```python
from build123d import *

# Parameters (mm, degrees)
SKETCH1_R           = 65
BOSS_EXTRUDE1_DEPTH = 30
SKETCH2_R           = 50
BOSS_EXTRUDE2_DEPTH = 250
FILLET1_R           = 10
FILLET2_R           = 10
SKETCH3_W           = 60
SKETCH3_H           = 35
BOSS_EXTRUDE3_DEPTH = 65
SKETCH4_R           = 13.35
CUT_EXTRUDE1_DEPTH  = 130
FILLET3_R           = 25


with BuildPart() as part:
    # Sketch1 → Boss-Extrude1 (new body)
    with BuildSketch(Plane(origin=(0, 0, 0), x_dir=(1, 0, 0), z_dir=(0, 1, 0))):
        with Locations(Location((0, 0, 0), (0, 0, 270))):
            Circle(SKETCH1_R)
    extrude(amount=BOSS_EXTRUDE1_DEPTH)

    # Sketch2 → Boss-Extrude2 (add)
    with BuildSketch(Plane.XZ):
        with Locations(Location((0, 0, 0), (0, 0, 90))):
            Circle(SKETCH2_R)
    extrude(amount=BOSS_EXTRUDE2_DEPTH)

    # Fillet1
    fillet1_edges = [part.edges().sort_by_distance(p)[0] for p in [
        (0, 0, -50),
    ]]
    fillet(fillet1_edges, radius=FILLET1_R)

    # Fillet2
    # the kernel refuses this fillet: 10 mm, written as the material it takes off along each edge
    with BuildSketch(Plane(origin=(0, 0, 0), x_dir=(0, 0, 1), z_dir=(-1, 0, 0))) as fillet2_piece_1:
        with BuildLine():
            CenterArc((55, 9.364916731), FILLET2_R, 284.477512186, 75.522487814)
            Line((65, 9.364916731), (66, 9.364916731))
            Line((66, 9.364916731), (66, 0))
            Line((66, 0), (65, -1))
            ThreePointArc((65, -1), (60, -1), (57.75, -1.285787471))
            Line((57.75, -1.285787471), (57.5, -0.317541634))
        make_face()
    revolve(axis=Axis((0, 0, 0), (0, 1, 0)), mode=Mode.SUBTRACT)

    # Sketch3 → Boss-Extrude3 (add, symmetric)
    with BuildSketch(Plane(origin=(0, 0, 0), x_dir=(0, 0, -1), z_dir=(1, 0, 0))):
        with Locations((0, 47.5)):
            Rectangle(SKETCH3_W, SKETCH3_H)
    extrude(amount=BOSS_EXTRUDE3_DEPTH, both=True)

    # Sketch4 → Cut-Extrude1 (cut)
    with BuildSketch(Plane(origin=(65, 0, 0), x_dir=(0, 0, -1), z_dir=(1, 0, 0))):
        with Locations((0, 47.897467929)):
            Circle(SKETCH4_R)
    extrude(amount=-CUT_EXTRUDE1_DEPTH, mode=Mode.SUBTRACT)

    # Fillet3
    fillet3_edges = [part.edges().sort_by_distance(p)[0] for p in [
        (0, 65, 30),
        (0, 65, -30),
    ]]
    fillet(fillet3_edges, radius=FILLET3_R)


solid = part.part
```
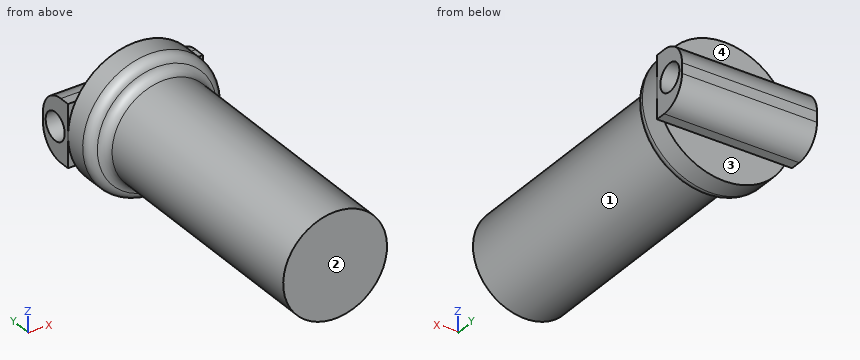
Verification items for the finished model (mm, model axes). Face numbers are marked on the shaded views. A direction names the side the tool comes from. Give positions to 0.01 mm unless a question says otherwise; leave off trailing zeros. Order: outer loops, then holes, each group sorted by start corner. A loop starts at its lowest first (then second) coordinate and runs counter-clockwise, first axis right, second up. Notation, with made-up numbers: M 45,84 L 71,84 A18 ccw 71,101 Z; hole C 78.5,-16 d1. An arc over 180 degrees is marked long. Return JSON: item names as keys, results as strings. Group by question number.
1) Section check B-B on y = -130. Record the cut outline in (x, z).
2) Scan lines: line 1 (Y direction, x = 26, z = 0); line 2 (Z direction, x = -55, y = 41.5); line 3 (Y direction, x = -31.5, z = 36.5). Record each from-to range of solid material in increasing order.
3) Access from +Z, -Z, +X, -X, +Y, -Y to the whole of each face (thin tool, end or side, straight path). Record for the marked faces 1, 2, 3 and 4.
4) Section check A-A on x = 0. Record the cut outline in (y, z), and give its area (3 significant figures).
5) Go/stop test with flat-tipped pins: pin 1 Ø3 at (x, y) = (-1.5, 34) entering from -Z; pin 2 Ø2 at (y, z) = (-39.5, -47) entering from -X; pin 3 Ø6 at (x, z) = (-63, -11.5) entering from -Y. Record where each tip stops, or that it passes through.
Answer block:
{
 "1": {"outline": "C 0,0 d100"},
 "2": {"line 1": "y = -250 to 34.55, 61.25 to 65", "line 2": "z = -29.95 to -11.72, 11.72 to 29.95", "line 3": "y = -250 to 30"},
 "3": {"face 1": "-Y", "face 2": "+Z, -Z, +X, -X, -Y", "face 3": "-Z, +X, -X, +Y", "face 4": "+Z, +X, -X, +Y"},
 "4": {"outline": "M -250,-50 L -10,-50 A10 cw -0.32,-57.5 A10 ccw 9.36,-65 L 30,-65 L 30,-30 L 40,-30 A25 ccw 65,-5 L 65,5 A25 ccw 40,30 L 30,30 L 30,65 L 9.36,65 A10 ccw -0.32,57.5 A10 cw -10,50 L -250,50 Z; hole C 47.9,0 d26.7", "area": "30,200 mm^2"},
 "5": {"pin 1": "stops at z = -30", "pin 2": "stops at x = -19.6", "pin 3": "stops at y = 1.4"}
}
